The listing builds one solid part. Answer for the finished solid, in the listing's coordinates (mm). A direction names the side the tool comes from. Give positions to 0.01 mm unless a question says otherwise; leave off trailing zeros. Loops run counter-clockwise (first coordinate to the right, second up) from the corner with the lowest first, then second, coordinate; pieces in that order, holes last. Notation, with made-up numbers: M 44,57.5 L 61,57.5 A21 cw 61,65.5 Z; hole C 79.5,-32 d4. An arc over 180 degrees is marked long. Return JSON: item names as keys, results as strings.
from build123d import *

# Parameters (mm, degrees)
F1_DEPTH = 7.62
F0_W     = 50.5
F0_H     = 50.5
F2_DEPTH = 2.54
F3_W     = 38.1
F3_H     = 38.1
F4_DEPTH = 5.08


# Not quite as in the source:
# - a feature names something its author has since deleted; it is built from what else it names


with BuildPart() as f1:
    # F0 (on Front) → F1 (new body)
    with BuildSketch(Plane.XZ):
        with BuildLine():
            Line((-3.3566042603, 23.25), (-23.25, 23.25))
            Line((-23.25, 23.25), (-23.25, 3.3541019662))
            ThreePointArc((-23.25, 3.3541019662), (-18.4128826929, 4.1079191813), (-15.75, 0))
            ThreePointArc((-15.75, 0), (-18.4128826929, -4.1079191813), (-23.25, -3.3541019662))
            Line((-23.25, -3.3541019662), (-23.25, -23.25))
            Line((-23.25, -23.25), (-3.3566042603, -23.25))
            ThreePointArc((-3.3566042603, -23.25), (-1.6039452654, -16.0483547827), (4.5, -20.2528))
            ThreePointArc((4.5, -20.2528), (4.2044452173, -21.8567452654), (3.3566042603, -23.25))
            Line((3.3566042603, -23.25), (23.25, -23.25))
            Line((23.25, -23.25), (23.25, -3.3566042603))
            ThreePointArc((23.25, -3.3566042603), (15.7528, 0), (23.25, 3.3566042603))
            Line((23.25, 3.3566042603), (23.25, 23.25))
            Line((23.25, 23.25), (3.3566042603, 23.25))
            ThreePointArc((3.3566042603, 23.25), (4.2044452173, 21.8567452654), (4.5, 20.2528))
            ThreePointArc((4.5, 20.2528), (-1.6039452654, 16.0483547827), (-3.3566042603, 23.25))
        make_face()
        with BuildLine():
            ThreePointArc((3.3566042603, 23.25), (0, 24.7528), (-3.3566042603, 23.25))
            Line((-3.3566042603, 23.25), (3.3566042603, 23.25))
        make_face()
        with BuildLine():
            Line((3.3566042603, 23.25), (-3.3566042603, 23.25))
            ThreePointArc((-3.3566042603, 23.25), (-1.6039452654, 16.0483547827), (4.5, 20.2528))
            ThreePointArc((4.5, 20.2528), (4.2044452173, 21.8567452654), (3.3566042603, 23.25))
        make_face()
        with BuildLine():
            ThreePointArc((-15.75, 0), (-18.4128826929, 4.1079191813), (-23.25, 3.3541019662))
            Line((-23.25, 3.3541019662), (-23.25, -3.3541019662))
            ThreePointArc((-23.25, -3.3541019662), (-18.4128826929, -4.1079191813), (-15.75, 0))
        make_face()
        with BuildLine():
            Line((-23.25, -3.3541019662), (-23.25, 3.3541019662))
            ThreePointArc((-23.25, 3.3541019662), (-24.75, 0), (-23.25, -3.3541019662))
        make_face()
        with BuildLine():
            ThreePointArc((4.5, -20.2528), (-1.6039452654, -16.0483547827), (-3.3566042603, -23.25))
            Line((-3.3566042603, -23.25), (3.3566042603, -23.25))
            ThreePointArc((3.3566042603, -23.25), (4.2044452173, -21.8567452654), (4.5, -20.2528))
        make_face()
        with BuildLine():
            Line((3.3566042603, -23.25), (-3.3566042603, -23.25))
            ThreePointArc((-3.3566042603, -23.25), (0, -24.7528), (3.3566042603, -23.25))
        make_face()
        with BuildLine():
            Line((23.25, -3.3566042603), (23.25, 3.3566042603))
            ThreePointArc((23.25, 3.3566042603), (15.7528, 0), (23.25, -3.3566042603))
        make_face()
        with BuildLine():
            ThreePointArc((24.7528, 0), (24.3599522981, 1.8388311505), (23.25, 3.3566042603))
            Line((23.25, 3.3566042603), (23.25, -3.3566042603))
            ThreePointArc((23.25, -3.3566042603), (24.3599522981, -1.8388311505), (24.7528, 0))
        make_face()
    extrude(amount=F1_DEPTH)

    # F0 (on Front) → F2 (join)
    with BuildSketch(Plane.XZ):
        Rectangle(F0_W, F0_H)
        with BuildLine():
            Line((-23.25, 3.3541019662), (-23.25, 23.25))
            Line((-23.25, 23.25), (-3.3566042603, 23.25))
            ThreePointArc((-3.3566042603, 23.25), (0, 24.7528), (3.3566042603, 23.25))
            Line((3.3566042603, 23.25), (23.25, 23.25))
            Line((23.25, 23.25), (23.25, 3.3566042603))
            ThreePointArc((23.25, 3.3566042603), (24.3599522981, 1.8388311505), (24.7528, 0))
            ThreePointArc((24.7528, 0), (24.3599522981, -1.8388311505), (23.25, -3.3566042603))
            Line((23.25, -3.3566042603), (23.25, -23.25))
            Line((23.25, -23.25), (3.3566042603, -23.25))
            ThreePointArc((3.3566042603, -23.25), (0, -24.7528), (-3.3566042603, -23.25))
            Line((-3.3566042603, -23.25), (-23.25, -23.25))
            Line((-23.25, -23.25), (-23.25, -3.3541019662))
            ThreePointArc((-23.25, -3.3541019662), (-24.75, 0), (-23.25, 3.3541019662))
        make_face(mode=Mode.SUBTRACT)
    extrude(amount=F2_DEPTH)

    # F3 (on face) → F4 (cut)
    with BuildSketch(Plane.XZ.offset(7.62)):
        Rectangle(F3_W, F3_H)
    extrude(amount=-F4_DEPTH, mode=Mode.SUBTRACT)


solid = f1.part
(1) Straight lines are drawn through the part: line 1 along X through (y, z) = (-4.75, -19); line 2 along Y through (x, z) = (-0.5, -2). For each, find the intervals that lie inside material, in ascending order.
Values follow:
{"line 1": "-23.25 to -19.05, 19.05 to 23.25", "line 2": "-2.54 to 0"}
(2) The part is cut by section B-B (x = 22). Determine the outline of the cut face in (y, z), and give its area (3 significant figures).
Values follow:
{"outline": "M -7.62,-23.25 L -2.54,-23.25 L -2.54,-25.25 L 0,-25.25 L 0,25.25 L -2.54,25.25 L -2.54,23.25 L -7.62,23.25 Z", "area": "364 mm²"}
(3) The part is cut by section D-D (z = -20.5). Determine the outline of the cut face in (x, y), and give its area (3 significant figures).
Values follow:
{"outline": "M -25.25,-2.54 L -23.25,-2.54 L -23.25,-7.62 L 23.25,-7.62 L 23.25,-2.54 L 25.25,-2.54 L 25.25,0 L -25.25,0 Z", "area": "364 mm²"}
(4) The part is cut by section A-A (z = 18). Determine the outline of the cut face in (x, y), and give its area (3 significant figures).
Values follow:
{"outline": "M -25.25,-2.54 L -23.25,-2.54 L -23.25,-7.62 L -19.05,-7.62 L -19.05,-2.54 L 19.05,-2.54 L 19.05,-7.62 L 23.25,-7.62 L 23.25,-2.54 L 25.25,-2.54 L 25.25,0 L -25.25,0 Z", "area": "171 mm²"}
(5) Given pin 1 (1.5 mm diameter, centred on x = -18, y = -6, fed in from -Z); pin 2 (4 mm diameter, centred on y = -5, z = -2, fed in from +X); pin 3 (2 mm diameter, centred on x = 17.5, y = -4.5, fed in from +Z), each flat-ended and moving along its own axis, determine where each tip first touches the part or whether it passes through.
Values follow:
{"pin 1": "z = -23.25", "pin 2": "x = 24.75", "pin 3": "z = 23.25"}
(6) The part is cut by section C-C (y = -3.5). Determine the outline of the cut face in (x, z).
Values follow:
{"outline": "M -23.25,-23.25 L -3.36,-23.25 A4.5 ccw 3.36,-23.25 L 23.25,-23.25 L 23.25,-3.36 A4.5 ccw 23.25,3.36 L 23.25,23.25 L 3.36,23.25 A4.5 ccw -3.36,23.25 L -23.25,23.25 L -23.25,3.35 A4.5 ccw -23.25,-3.35 Z; hole M -19.05,-19.05 L 19.05,-19.05 L 19.05,19.05 L -19.05,19.05 Z"}
(7) Determine the mould class of faces 1 (the cylindrical face through (0.053, -5.044, 24.752)), 2 (the flat face through (0, -5, -19.05)), 3 (the flat face through (13, -5, 23.25)), 4 (the flat face through (-23.25, -5, 13)) for opening direction X: released by +X, released by -X, zero draft, split by the parting line, or undercut.
Values follow:
{"face 1": "split by the parting line", "face 2": "undercut", "face 3": "zero draft", "face 4": "released by -X"}
(8) A tool of negligible diameter and unlimited length cuts with its end or side. For faces 5 (the cylindrical face through (-0.053, -5.044, -24.752)), 6 (the cylindrical face through (-24.75, -5.04, 0.05)), 7 (the flat face through (-19.05, -5, 0)), 8 (the flat face through (-13, -5, -23.25)), 9 (the flat face through (-13, -5, 23.25)), from which of +Z, -Z, +X, -X, +Y, -Y can it reach the whole face along a straight path? Write none if from no direction.
Values follow:
{"face 5": "-Z, -Y", "face 6": "-X, -Y", "face 7": "-Y", "face 8": "-Z, -X, -Y", "face 9": "+Z, -X, -Y"}
